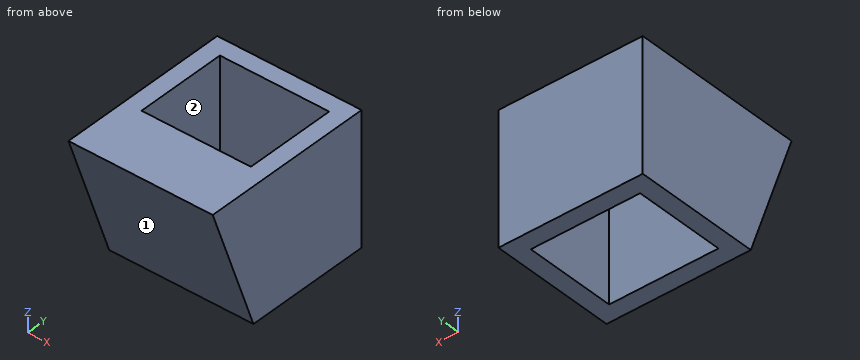
```python
from build123d import *

# Parameters (mm, degrees)
SKETCH1_W           = 16.5
SKETCH1_H           = 14.5
SKETCH1_W_2         = 12.5
SKETCH1_H_2         = 10.5
BOSS_EXTRUDE1_DEPTH = 15
BOSS_EXTRUDE2_DEPTH = 16.5


with BuildPart() as part:
    # Sketch1 → Boss-Extrude1 (new body)
    with BuildSketch(Plane.XY):
        with Locations((6.25, -5.25)):
            Rectangle(SKETCH1_W, SKETCH1_H)
        with Locations((6.25, -5.25)):
            Rectangle(SKETCH1_W_2, SKETCH1_H_2, mode=Mode.SUBTRACT)
    extrude(amount=BOSS_EXTRUDE1_DEPTH)

    # Sketch2 → Boss-Extrude2 (add)
    with BuildSketch(Plane.ZY.offset(2)):
        Polygon((0, -12.5), (15, -17.959553514), (15, -12.5), align=None)
    extrude(amount=-BOSS_EXTRUDE2_DEPTH)


solid = part.part
```
Build history of the part. All positions in model axes, mm. Face numbers are marked on the shaded views. A direction names the side the tool comes from. Give positions to 0.01 mm unless a question says otherwise; leave off trailing zeros. Order: outer loops, then holes, each group sorted by start corner. A loop starts at its lowest first (then second) coordinate and runs counter-clockwise, first axis right, second up. Notation, with made-up numbers: M 66,12 L 72,12 A20 cw 72,38 Z; hole C 87,-30.75 d7. An arc over 180 degrees is marked long. Return JSON: item names as keys, results as strings.
Q1. Band-saw the part on A-A (x = 10.5). Give the cut face in (y, z).
Answer list:
{"outline": "M -17.96,15 L -12.5,0 L -10.5,0 L -10.5,15 Z; M 0,0 L 2,0 L 2,15 L 0,15 Z"}
Q2. 3-axis set-ups, long thin cutter, end or side, ignore diameter. For the marked faces 1 and 2: which of +Z, -Z, +X, -X, +Y, -Y reach the whole face in a straight line?
Answer list:
{"face 1": "-Z, +X, -X, -Y", "face 2": "+Z, -Z"}
Q3. Wall check: probe 1 along X at (y, z) = (-1, 2.25); probe 2 along Y at (x, z) = (4.5, 14.25); probe 3 along Y at (x, z) = (5.75, 7). Give the ranges that are in metal, low to high. Write a range as from..to.
Answer list:
{"probe 1": "x = -2..0, 12.5..14.5", "probe 2": "y = -17.69..-10.5, 0..2", "probe 3": "y = -15.05..-10.5, 0..2"}
Q4. Flat gauge pins, fed straight in: pin 1 (1.5 mm diameter, centred on x = 3.5, y = -2, fed in from +Z); pin 2 (3 mm diameter, centred on x = 3.5, z = 3.5, fed in from -Y); pin 3 (4 mm diameter, centred on x = 8, z = 6.5, fed in from -Y). Where does each tip first touch, or does it go through?
Answer list:
{"pin 1": "passes through", "pin 2": "stops at y = -14.32", "pin 3": "stops at y = -15.59"}
Q5. Band-saw the part on D-D (z = 4). Give the cut face in (x, y).
Answer list:
{"outline": "M -2,-13.96 L 14.5,-13.96 L 14.5,2 L -2,2 Z; hole M 0,-10.5 L 12.5,-10.5 L 12.5,0 L 0,0 Z"}
Q6. Band-saw the part on C-C (z = 12.5). Give the cut face in (x, y).
Answer list:
{"outline": "M -2,-17.05 L 14.5,-17.05 L 14.5,2 L -2,2 Z; hole M 0,-10.5 L 12.5,-10.5 L 12.5,0 L 0,0 Z"}
Q7. Band-saw the part on B-B (y = -9.75). Give the cut face in (x, z), then the cut area to 3 significant figures.
Answer list:
{"outline": "M -2,0 L 0,0 L 0,15 L -2,15 Z; M 12.5,0 L 14.5,0 L 14.5,15 L 12.5,15 Z", "area": "60.0 mm^2"}
